Geometry: final body of the model. Coordinates: model frame, mm. A direction names the side the tool comes from. Give positions to 0.01 mm unless a question says otherwise; leave off trailing zeros. Loops run counter-clockwise (first coordinate to the right, second up) from the corner with the lowest first, then second, coordinate; pieces in that order, holes last.
Autodesk Inventor part; units mm, degrees
ref_plane "YZ Plane" through (0, 0, 0) normal (1, 0, 0) x (0, 1, 0)
ref_plane "XZ Plane" through (0, 0, 0) normal (0, 1, 0) x (-1, 0, 0)
ref_plane "XY Plane" through (0, 0, 0) normal (0, 0, 1) x (1, 0, 0)
sketch "草圖1" plane through (0, 0, 0) normal (0, 1, 0) x (-1, 0, 0)
  line L0 (0, 0) -> (-50, 0)
  line L1 (-50, 0) -> (-50, -40)
  line L2 (-50, -40) -> (0, -40)
  line L3 (0, -40) -> (0, 0)
  dimension "d0" = 50
  dimension "d1" = 40
extrude "擠出1" add sketch "草圖1" along normal blind 10
sketch "草圖2" plane through (0, 0, -40) normal (-1, 0, 0) x (0, 0, 1)
  line L0 (0, 0) -> (0, 10)
  line L1 (0, 10) -> (40, 10)
  line L2 (40, 10) -> (40, 20)
  line L3 (40, 20) -> (0, 20)
  line L4 (0, 20) -> (0, 10)
  line L5 (0, 20) -> (30, 20)
  line L6 (30, 20) -> (30, 30)
  line L7 (30, 30) -> (0, 30)
  line L8 (0, 30) -> (0, 20)
  point P0 (40, 0)
  dimension "d4" = 30
  dimension "d5" = 40
  dimension "d6" = 10
  dimension "d7" = 10
extrude "擠出2" add sketch "草圖2" against normal blind 10
fillet "圓角1" radius 20 2 edges at (50, 5, 0) (50, 5, -40)
hole "孔1" at (30, 0, -20) direction (0, 1, 0) diameter 20 depth 10 tip angle 118
properties part number "35"
Item 1: Section query C-C on y = 21.75. Return loops of the section in (x, z), plus the area to 3 significant figures.
Values follow:
outline: (0, -40) - (10, -40) - (10, -10) - (0, -10) - close
area: 300 mm2
Item 2: Section query A-A on z = -18. Return loops of the section in (x, y).
Values follow:
outline: (0, 0) - (20.2, 0) - (20.2, 10) - (10, 10) - (10, 30) - (0, 30) - close; (39.8, 0) - (49.9, 0) - (49.9, 10) - (39.8, 10) - close
Item 3: Section query D-D on x = 16. Return loops of the section in (y, z), plus the area to 3 significant figures.
Values follow:
outline: (0, -40) - (10, -40) - (10, 0) - (0, 0) - close
area: 400 mm2
Item 4: Ray query, probe 1 along X at (y, z) = (5, -20); probe 2 along Z at (x, y) = (30, 2.75); probe 3 along Y at (x, z) = (11, -11). Return the intervals inside material, ascending.
Values follow:
probe 1: x = 0 to 20, 40 to 50
probe 2: z = -40 to -30, -10 to 0
probe 3: y = 0 to 10
Item 5: Section query B-B on x = 32. Return loops of the section in (y, z), plus the area to 3 significant figures.
Values follow:
outline: (0, -39.9) - (10, -39.9) - (10, -29.8) - (0, -29.8) - close; (0, -10.2) - (10, -10.2) - (10, -0.1) - (0, -0.1) - close
area: 202 mm2
Item 6: Draft query along X for faces 4 (the face through (10, 20, -20)), 5 (the face through (38.872, 5.07, -24.614)), 6 (the face through (5, 20, -5)). Return one class per face: +X half, -X half, draft (parallel to the pull), parting line (faces both ways), or undercut.
Values follow:
face 4: +X half
face 5: undercut
face 6: draft
Item 7: Set-up query: faces 1 (the face through (5, 25, -10)), 2 (the face through (11, 8, 0)), 3 (the face through (17, 10, -20)). Return all of +Z, -Z, +X, -X, +Y, -Y with unobstructed straight access to the full face (end or side cutting, diameter ignored); none if empty.
Values follow:
face 1: +Z, +X, -X, +Y
face 2: +Z, +X, -X, +Y, -Y
face 3: +Z, -Z, +X, +Y
Item 8: Pin query (flat end, axial travel): pin 1 (6 mm diameter, centred on y = 8.5, z = -34, fed in from -X); pin 2 (5 mm diameter, centred on x = 6.5, z = -2.5, fed in from +Y); pin 3 (6 mm diameter, centred on y = 24, z = -14.5, fed in from +X); pin 4 (3 mm diameter, centred on x = 3.5, y = 24.5, fed in from +Z). Return the tip coordinate at first contact, or that it passes through.
Values follow:
pin 1: stops at x = 0
pin 2: stops at y = 20
pin 3: stops at x = 10
pin 4: stops at z = -10
